from build123d import *

# Parameters (mm, degrees)
F1_DEPTH = 60
F2_R     = 6
F3_DEPTH = 25
F4_R     = 6
F4_R_2   = 4
F5_DEPTH = 155.501


with BuildPart() as f1:
    # F0 (on Front) → F1 (new body)
    with BuildSketch(Plane.XZ):
        Polygon((104.208015, 89.68718), (-95.791985, 89.68718), (-95.791985, 84.68718), (-51.291985, 84.68718), (-51.291985, -110.31282), (-46.291985, -110.31282), (-46.291985, 84.68718), (54.708015, 84.68718), (54.708015, -110.31282), (59.708015, -110.31282), (59.708015, 84.68718), (104.208015, 84.68718), align=None)
    extrude(amount=F1_DEPTH)

    # F2 (on face) → F3 (cut)
    with BuildSketch(Plane.XY.offset(89.68718)):
        with Locations((-83.791985, -12)):
            Circle(F2_R)
        with Locations((83.791985, -12)):
            Circle(F2_R)
        with Locations((-83.791985, -48)):
            Circle(F2_R)
        with Locations((83.791985, -48)):
            Circle(F2_R)
    extrude(amount=-F3_DEPTH, mode=Mode.SUBTRACT)

    # F4 (on face) → F5 (cut, through all)
    with BuildSketch(Plane(origin=(-51.291985, 0, 0), x_dir=(0, -1, 0), z_dir=(-1, 0, 0))):
        with Locations((30, 54.878019)):
            Circle(F4_R)
        with Locations((30, -86.190678)):
            Circle(F4_R)
        with Locations((30, -6.819744)):
            Circle(F4_R_2)
        with Locations((14.702255, -39.625864)):
            Circle(F4_R_2)
        with Locations((45.297745, 25.986376)):
            Circle(F4_R_2)
        with Locations((47.644541, -73.885843)):
            Circle(F4_R_2)
    extrude(amount=-F5_DEPTH, mode=Mode.SUBTRACT)


solid = f1.part
Design review of the part built by this model. Coordinates are the model's own, in mm. A direction names the side the tool comes from. Coordinates: 2 decimals unless noted, no trailing zeros. Write each loop counter-clockwise with the first axis right and the second up, starting at its lowest first coordinate (ties: lowest second). Pieces come first, ordered by that corner, then holes. Notation, with made-up numbers: (81.25, 61.5) -> (125.25, 61.5) arc R17 ccw to (125.25, 91.5) -> close; hole circle Ø3 at (-16, 88.5). An arc over 180 degrees is marked (long way). Write each question's results on one line, items separated by ' | '. Start each with the question number.
(1) Take a section at C-C on x = 81. Write out the cut boundary in (y, z), and give its area (3 significant figures).
(2) For line 1 along Z through (x, y) = (57.9, -30); line 2 along X through (y, z) = (-8.5, -80.5); line 3 along Z through (x, y) = (-47, -14.5), list the stretches that pass through material, from the lowest coordinate up. Write a range as from..to.
(3) The part is to be moulded in two halves that separate along X. For faces 3 (the face through (57.173, -18.518, -38.424)), 4 (the face through (-89.786, -47.736, 87.222)), 5 (the face through (-51.292, -30, -11)), say which applies: pulls with the +X half, pulls with the -X half, needs draft (parallel to the pull), parting line crosses it, or undercut.
(4) Take a section at B-B on y = -30. Give the number of separate pieces and of enclosed holes in the cut face, and give its area (3 significant figures).
(5) Take a section at A-A on z = -51. Write out the cut boundary in (x, y), and give its area (3 significant figures).
(6) Take a section at D-D on x = -54. Write out the cut boundary in (y, z).
(7) Clearance check with flat-ended pins moving along their axes: P1, Ø6.5, axis at y = -30, z = -6.82, coming from the -X side; P2, Ø6, axis at y = -33, z = 23, coming from the -X side; P3, Ø5, axis at x = 36.5, y = -28.5, coming from the -Z side; P4, Ø2, axis at y = -34, z = 47, coming from the +X side. State where each tip first meets the part, or that it passes through.
(8) Tool access review of faces 1 (the face through (4, -30, 84.687)), 2 (the face through (-48, 0, 20)): name each direction out of +Z, -Z, +X, -X, +Y, -Y from which nothing blocks a thin tool from reaching the whole face with its end or side.
Results found:
1) outline: (-60, 84.69) -> (-53.31, 84.69) -> (-53.31, 89.69) -> (-60, 89.69) -> close; (-42.69, 84.69) -> (-17.31, 84.69) -> (-17.31, 89.69) -> (-42.69, 89.69) -> close; (-6.69, 84.69) -> (0, 84.69) -> (0, 89.69) -> (-6.69, 89.69) -> close | area: 194 mm2
2) line 1: z = -110.31..-92.19, -80.19..-10.82, -2.82..48.88, 60.88..89.69 | line 2: x = -51.29..-46.29, 54.71..59.71 | line 3: z = -110.31..-43.62, -35.63..89.69
3) face 3: needs draft | face 4: undercut | face 5: pulls with the -X half
4) separate pieces: 7 | enclosed holes: 0 | area: 2,630 mm2
5) outline: (-51.29, -60) -> (-46.29, -60) -> (-46.29, 0) -> (-51.29, 0) -> close; (54.71, -60) -> (59.71, -60) -> (59.71, 0) -> (54.71, 0) -> close | area: 600 mm2
6) outline: (-60, 84.69) -> (0, 84.69) -> (0, 89.69) -> (-60, 89.69) -> close
7) P1: passes through | P2: stops at x = -51.29 | P3: stops at z = 84.69 | P4: stops at x = 59.71
8) face 1: -Z, +Y, -Y | face 2: +Z, -Z, +X, -X, +Y
